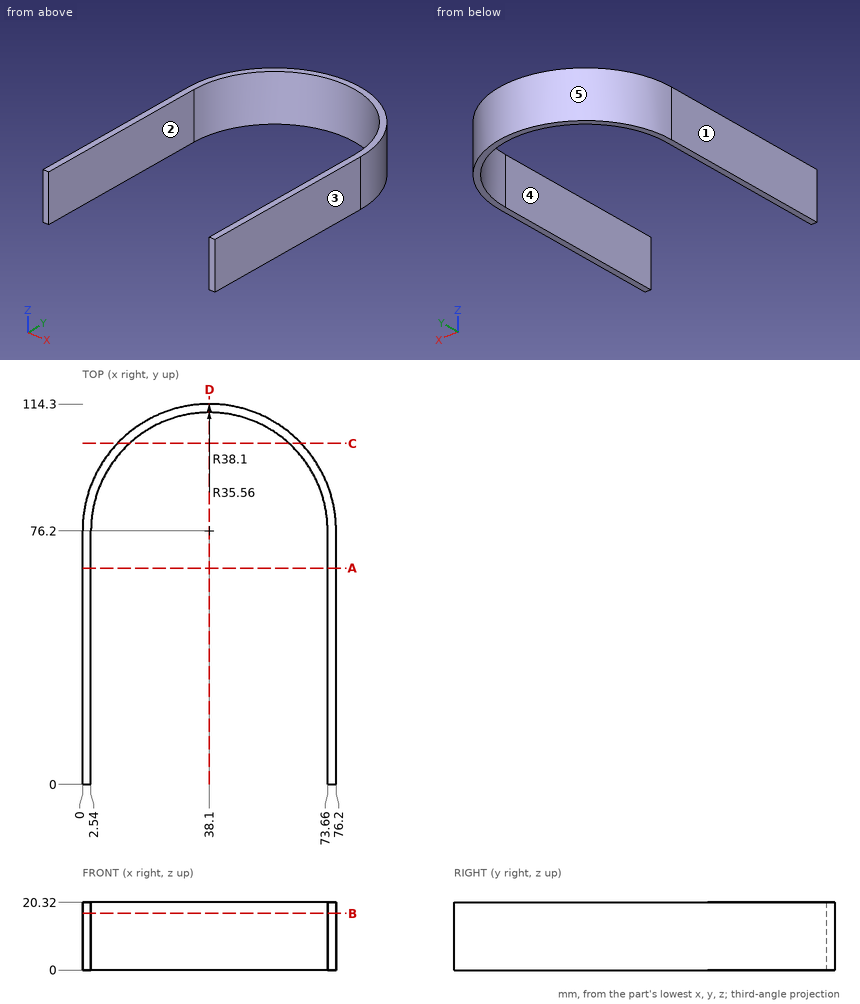
Could you check a few things on this drawing? It's one solid part, dimensions in mm from its lowest x, y, z. A direction names the side the tool comes from. Coordinates: 2 decimals unless noted, no trailing zeros. Write each loop counter-clockwise with the first axis right and the second up, starting at its lowest first coordinate (ties: lowest second). Pieces come first, ordered by that corner, then holes. Notation, with made-up numbers: (53.5, 59.5) - (108.5, 59.5) arc R6 cw to (108.5, 63.5) - close; hole circle Ø5 at (42.25, 79.5). An arc over 180 degrees is marked (long way). Return JSON: item names as keys, results as strings. Group by question number.
Item 1: If we section it at D-D (x = 38.1): Write out the boundary of the cut face in (y, z).
Item 2: Which directions (+Z, -Z, +X, -X, +Y, -Y) give clear straight access to the entire face, cutting with the end or side of a thin tool? Please do the marked faces 1 and 2.
Item 3: I'm going to push flat-ended pins straight in: pin 1 Ø12 at (x, z) = (42, 17) entering from -Y; pin 2 Ø1 at (y, z) = (87.5, 11.5) entering from -X; pin 3 Ø4 at (x, z) = (48.5, 14) entering from -Y. Where does each tip first touch, or does it pass through?
Item 4: If we section it at C-C (y = 102.5): Write out the boundary of the cut face in (x, z).
Item 5: Please list where these lines run through material, in increasing order: probe 1 along X at (y, z) = (57, 15); probe 2 along X at (y, z) = (92, 5.75); probe 3 along Y at (x, z) = (12, 6.5).
Item 6: We'd pull the mould along X, two halves only. Please class the marked faces 3, 4 and 5: pulls with the +X half, pulls with the -X half, needs draft (parallel to the pull), parting line crosses it, or undercut.
Item 7: If we section it at A-A (y = 65): Write out the boundary of the cut face in (x, z), then the cut area to 3 significant figures.
Item 8: If we section it at B-B (z = 17): Write out the boundary of the cut face in (x, y), then the cut area to 3 significant figures.
Return value:
{
 "1": {"outline": "(111.76, 0) - (114.3, 0) - (114.3, 20.32) - (111.76, 20.32) - close"},
 "2": {"face 1": "+Z, -Z, -X, +Y, -Y", "face 2": "+Z, -Z, -Y"},
 "3": {"pin 1": "stops at y = 110.35", "pin 2": "stops at x = 1.56", "pin 3": "stops at y = 109.53"},
 "4": {"outline": "(10.53, 0) - (14.17, 0) - (14.17, 20.32) - (10.53, 20.32) - close; (62.03, 0) - (65.67, 0) - (65.67, 20.32) - (62.03, 20.32) - close"},
 "5": {"probe 1": "x = 0 to 2.54, 73.66 to 76.2", "probe 2": "x = 3.43 to 6.24, 69.96 to 72.77", "probe 3": "y = 100.35 to 103.96"},
 "6": {"face 3": "pulls with the +X half", "face 4": "undercut", "face 5": "parting line crosses it"},
 "7": {"outline": "(0, 0) - (2.54, 0) - (2.54, 20.32) - (0, 20.32) - close; (73.66, 0) - (76.2, 0) - (76.2, 20.32) - (73.66, 20.32) - close", "area": "103 mm^2"},
 "8": {"outline": "(0, 0) - (2.54, 0) - (2.54, 76.2) arc R35.56 cw to (73.66, 76.2) - (73.66, 0) - (76.2, 0) - (76.2, 76.2) arc R38.1 ccw to (0, 76.2) - close", "area": "681 mm^2"}
}
